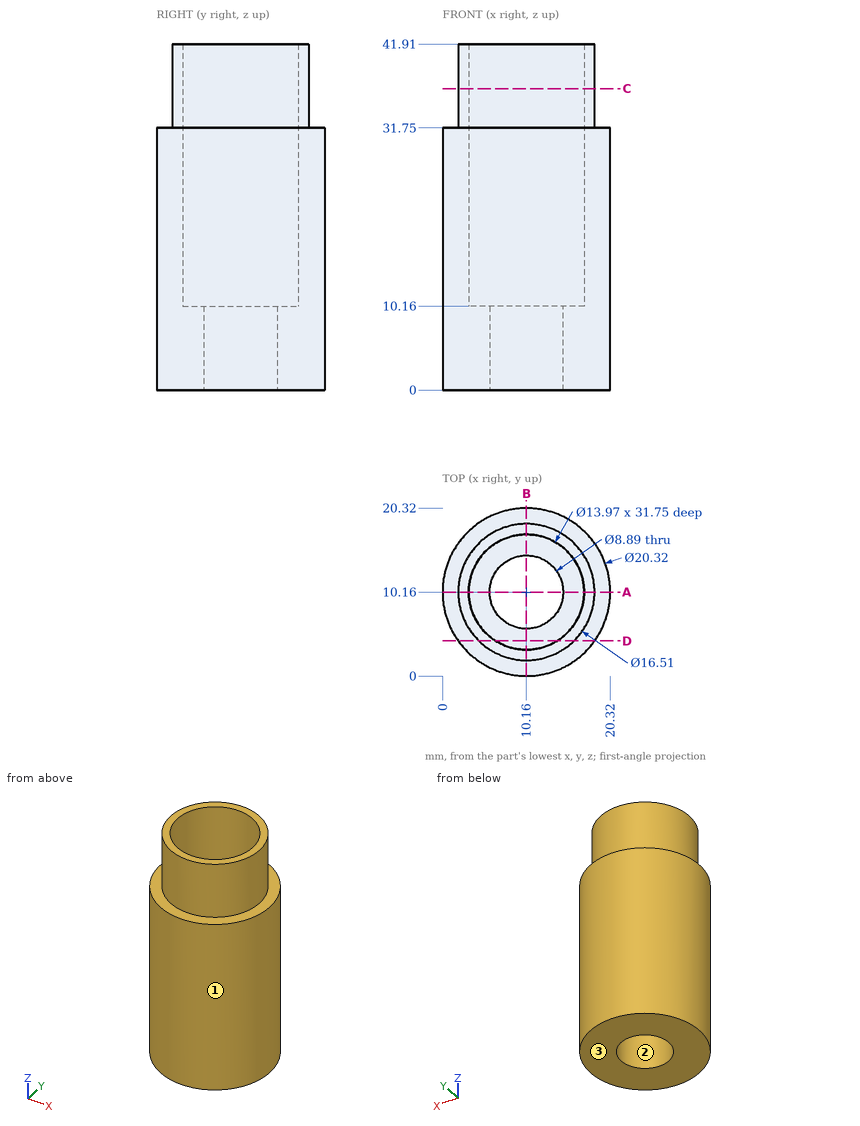
Geometry: see drawing. Coordinates: mm, zero at the bounding-box minimum. Round coordinates to 2 decimals unless told otherwise and drop trailing zeros. Order: outer loops, then holes, each group sorted by start corner. A loop starts at its lowest first (then second) coordinate and runs counter-clockwise, first axis right, second up. Notation, with made-up numbers: (38.25, -0.5) -> (78.25, -0.5) arc R20 cw to (78.25, 20.5) -> close; hole circle Ø7 at (0, 41). An arc over 180 degrees is marked (long way). Answer as CSV lines item,"result".
Item 1: Pin query (flat end, axial travel): pin 1 Ø2 at (y, z) = (3.5, 7) entering from +X; pin 2 Ø6 at (y, z) = (11, 15) entering from -X; pin 3 Ø2 at (y, z) = (3.5, 9.5) entering from -X; pin 4 Ø1 at (x, z) = (6, 19.5) entering from +Y. Return the tip coordinate at first contact, or that it passes through.
A:
pin 1,"x = 18.6"
pin 2,"x = 0"
pin 3,"x = 1.72"
pin 4,"y = 19.64"
Item 2: Section D-D, the plane y = 4.25. Return loops of the section in (x, z).
A:
outline,"(1.9, 0) -> (18.42, 0) -> (18.42, 31.75) -> (15.92, 31.75) -> (15.92, 41.91) -> (13.88, 41.91) -> (13.88, 10.16) -> (6.44, 10.16) -> (6.44, 41.91) -> (4.4, 41.91) -> (4.4, 31.75) -> (1.9, 31.75) -> close"
Item 3: Pull-direction query (Y, two-part tool) for the marked faces 1, 2 and 3; classes: pulls with the +Y half, pulls with the -Y half, needs draft (parallel to the pull), parting line crosses it, or undercut.
A:
face 1,"parting line crosses it"
face 2,"undercut"
face 3,"needs draft"
Item 4: Section A-A, the plane y = 10.16. Return loops of the section in (x, z) (3 decimals), plus the area to 3 significant figures.
A:
outline,"(0, 0) -> (5.715, 0) -> (5.715, 10.16) -> (3.175, 10.16) -> (3.175, 41.91) -> (1.905, 41.91) -> (1.905, 31.75) -> (0, 31.75) -> close; (14.605, 0) -> (20.32, 0) -> (20.32, 31.75) -> (18.415, 31.75) -> (18.415, 41.91) -> (17.145, 41.91) -> (17.145, 10.16) -> (14.605, 10.16) -> close"
area,"279 mm²"
Item 5: Line query: L1, parallel to Y at x = 10.16, z = 24 (3 decimals); L2, parallel to Z at x = 5.5, y = 10; L3, parallel to Y at x = 10.16, z = 5.5 (3 decimals). Output: solid intervals per line, ascending.
A:
L1,"0 to 3.175, 17.145 to 20.32"
L2,"0 to 10.16"
L3,"0 to 5.715, 14.605 to 20.32"
Item 6: Section C-C, the plane z = 36.5. Return loops of the section in (x, y) (3 decimals), plus the area to 3 significant figures.
A:
outline,"circle Ø16.51 at (10.16, 10.16); hole circle Ø13.97 at (10.16, 10.16)"
area,"60.8 mm²"
